```python
from build123d import *

# Parameters (mm, degrees)
CORNERBOSS_EXTRUDE1_DEPTH               = 20
SHELL1_T                                = -3
PADSKETCH1_R                            = 5
PADSKETCH1_R_2                          = 12
PADBOSS_EXTRUDE1_DEPTH                  = 10
STEPPERSHAFTCUT_SKETCH3_R               = 5.1
STEPPERSHAFTCUT_SKETCH3_R_2             = 2
STEPPERSHAFTCUT_EXTRUDE1_DEPTH          = 262.09193783
THREADEDNUTMOUNTHOLESSKETCH5_R          = 2
THREADEDNUTMOUNTHOLESCUT_EXTRUDE2_DEPTH = 10
TOPPEGHOLESKETCH4_W                     = 10
TOPPEGHOLESKETCH4_H                     = 14
TOPPEGHOLECUT_EXTRUDE2_DEPTH            = 3
BLPEGSKETCH5_W                          = 9.8
BLPEGSKETCH5_H                          = 13.9
BLPEGBOSS_EXTRUDE3_DEPTH                = 3.1
BLPEGCAPSKETCH6_W                       = 16
BLPEGCAPSKETCH6_H                       = 17
BLPEGCAPBOSS_EXTRUDE4_DEPTH             = 3
BEDCENTERPEGHOLECUTSKETCH1_W            = 10
BEDCENTERPEGHOLECUTSKETCH1_H            = 14
BEDCENTERPEGHOLECUT_EXTRUDE1_DEPTH      = 3


with BuildPart() as part:
    # CornerrSketch1 → CornerBoss-Extrude1 (new body)
    with BuildSketch(Plane(origin=(0, 0, 0), x_dir=(1, 0, 0), z_dir=(0, 1, 0))):
        with BuildLine():
            Line((0, 0), (0, 80))
            Line((0, 80), (70, 80))
            Line((70, 80), (70, 220))
            Line((70, 220), (140, 220))
            Line((140, 220), (140, -45.825))
            ThreePointArc((140, -45.825), (123, -62.825), (106, -45.825))
            Line((106, -45.825), (106, 0))
            Line((106, 0), (0, 0))
        make_face()
    extrude(amount=CORNERBOSS_EXTRUDE1_DEPTH)

    # Shell1
    shell1_openings = [part.faces().sort_by_distance(p)[0] for p in [
        (89.539211683, 0, -80.750143578),
    ]]
    offset(amount=SHELL1_T, openings=shell1_openings, kind=Kind.INTERSECTION)

    # PadSketch1 → PadBoss-Extrude1 (add)
    with BuildSketch(Plane.XZ.offset(-17)):
        with Locations(Location((99, -17, 0), (0, 0, 90))):
            Circle(PADSKETCH1_R)
        with Locations(Location((123, 45.825, 0), (0, 0, 90))):
            Circle(PADSKETCH1_R_2)
    extrude(amount=PADBOSS_EXTRUDE1_DEPTH)

    # StepperShaftCut-Sketch3 → StepperShaftCut-Extrude1 (cut, through all)
    with BuildSketch(Plane.XZ.offset(-7)):
        with Locations(Location((123, 45.825, 0), (0, 0, 270))):
            Circle(STEPPERSHAFTCUT_SKETCH3_R)
        with Locations(Location((99, -17, 0), (0, 0, 270))):
            Circle(STEPPERSHAFTCUT_SKETCH3_R_2)
    extrude(amount=-STEPPERSHAFTCUT_EXTRUDE1_DEPTH, mode=Mode.SUBTRACT)

    # ThreadedNutMountHolesSketch5 → ThreadedNutMountHolesCut-Extrude2 (cut)
    with BuildSketch(Plane.XZ.offset(-7)):
        with Locations(Location((123, 53.825, 0), (0, 0, 270))):
            Circle(THREADEDNUTMOUNTHOLESSKETCH5_R)
        with Locations(Location((131, 45.825, 0), (0, 0, 270))):
            Circle(THREADEDNUTMOUNTHOLESSKETCH5_R)
        with Locations(Location((115, 45.825, 0), (0, 0, 270))):
            Circle(THREADEDNUTMOUNTHOLESSKETCH5_R)
        with Locations(Location((123, 37.825, 0), (0, 0, 270))):
            Circle(THREADEDNUTMOUNTHOLESSKETCH5_R)
    extrude(amount=-THREADEDNUTMOUNTHOLESCUT_EXTRUDE2_DEPTH, mode=Mode.SUBTRACT)

    # TopPegHoleSketch4 → TopPegHoleCut-Extrude2 (cut)
    with BuildSketch(Plane(origin=(0, 0, -220), x_dir=(-1, 0, 0), z_dir=(0, 0, -1))):
        with Locations((-125, 7)):
            Rectangle(TOPPEGHOLESKETCH4_W, TOPPEGHOLESKETCH4_H)
    extrude(amount=-TOPPEGHOLECUT_EXTRUDE2_DEPTH, mode=Mode.SUBTRACT)

    # BLPegSketch5 → BLPegBoss-Extrude3 (add)
    with BuildSketch(Plane.ZY):
        with Locations((-15, 6.95)):
            Rectangle(BLPEGSKETCH5_W, BLPEGSKETCH5_H)
    extrude(amount=BLPEGBOSS_EXTRUDE3_DEPTH)

    # BLPegCapSketch6 → BLPegCapBoss-Extrude4 (add)
    with BuildSketch(Plane.ZY.offset(3.1)):
        with Locations((-14.9, 8.5)):
            Rectangle(BLPEGCAPSKETCH6_W, BLPEGCAPSKETCH6_H)
    extrude(amount=BLPEGCAPBOSS_EXTRUDE4_DEPTH)

    # BedCenterPegHoleCutSketch1 → BedCenterPegHoleCut-Extrude1 (cut)
    with BuildSketch(Plane.ZY.offset(-70)):
        with Locations((-185, 7)):
            Rectangle(BEDCENTERPEGHOLECUTSKETCH1_W, BEDCENTERPEGHOLECUTSKETCH1_H)
    extrude(amount=-BEDCENTERPEGHOLECUT_EXTRUDE1_DEPTH, mode=Mode.SUBTRACT)


solid = part.part
```
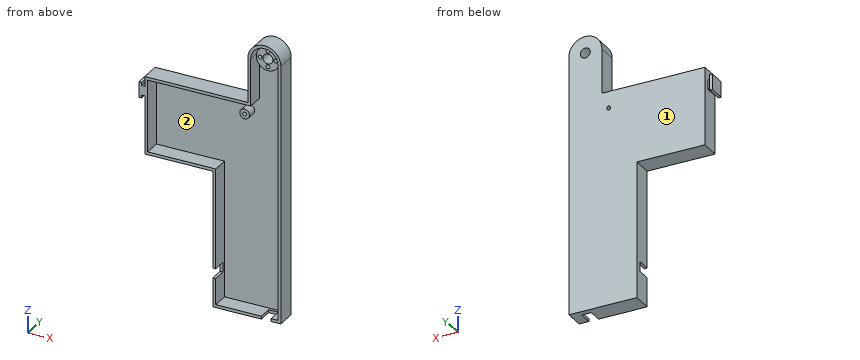
The model under review builds one solid part; all positions refer to its coordinate system, in mm. Face numbers are marked on the shaded views. A direction names the side the tool comes from. Round coordinates to 2 decimals unless told otherwise and drop trailing zeros. Order: outer loops, then holes, each group sorted by start corner. A loop starts at its lowest first (then second) coordinate and runs counter-clockwise, first axis right, second up. Notation, with made-up numbers: (26, -11.75) -> (38, -11.75) arc R19 ccw to (38, 6.25) -> close; hole circle Ø5 at (-36, 18.25). An arc over 180 degrees is marked (long way). One line per item, written item: value. Start each with the question number.
Q1. Clearance check with flat-ended pins moving along their axes: pin 1 Ø5 at (x, y) = (35.5, 9) entering from +Z; pin 2 Ø4 at (x, y) = (11, 15.5) entering from -Z; pin 3 Ø8.5 at (y, z) = (5.5, -127.5) entering from -X; pin 4 Ø6 at (x, y) = (121, 10) entering from +Z (3 decimals). State where each tip first meets the part, or that it passes through.
Q2. Wall thickness on line 1 (X direction, y = 7.5, z = 45.5); line 2 (X direction, y = 2.25, z = -23); line 3 (X direction, y = 10, z = -191): over which ranges is each line inside the solid? List them lowest first.
Q3. Machinability: for the marked faces 1 and 2, which of the approach directions +Z, -Z, +X, -X, +Y, -Y give a long, thin tool a straight path to every point of the face, cutting with its end or side? Answer none if there is none.
Q4. Take a section at A-A (z = -26.5). Write out the cut boundary in (x, y).
Q5. Take a section at B-B (x = 76.5). Write out the cut boundary in (y, z), and give its area (3 significant figures).
Reported:
1. pin 1: stops at z = 0
1. pin 2: stops at z = -80
1. pin 3: stops at x = 70
1. pin 4: stops at z = 62.825
2. line 1: x = 106 to 109, 111 to 113.03, 116.97 to 117.91, 128.09 to 129.03, 132.97 to 135, 137 to 140
2. line 2: x = 0 to 3, 137 to 140
2. line 3: x = 70 to 73, 137 to 140
3. face 1: +Z, -Z, +X, -X, +Y
3. face 2: -Y
4. outline: (0, 0) -> (3, 0) -> (3, 17) -> (137, 17) -> (137, 0) -> (140, 0) -> (140, 20) -> (0, 20) -> close
5. outline: (0, -220) -> (20, -220) -> (20, 0) -> (0, 0) -> (0, -3) -> (17, -3) -> (17, -217) -> (0, -217) -> close
5. area: 762 mm2
